Can you work these out from the model? Positions are in its coordinate system, mm. Face numbers are marked on the shaded views. A direction names the side the tool comes from. Give positions to 0.01 mm unless a question says otherwise; leave off trailing zeros. Order: outer loops, then holes, each group sorted by start corner. A loop starts at its lowest first (then second) coordinate and runs counter-clockwise, first axis right, second up. Notation, with made-up numbers: (-20.75, -23.75) - (1.25, -23.75) arc R23 ccw to (1.25, 11.25) - close; hole circle Ø1 at (-22.75, -39.5). An arc over 180 degrees is marked (long way). Use one line per item in the form item = value. Start each with the question number.
1) Please list where these lines run through material, in increasing order: probe 1 along Z at (x, y) = (17, 14); probe 2 along X at (y, z) = (9.5, 20); probe 3 along Z at (x, y) = (18.25, 18).
2) Suppose I cut it at B-B, the plane y = 11.25. Write out the boundary of the cut face in (x, z), and give its area (3 significant figures).
3) For pin 1 (3 mm diameter, centred on x = 12.5, y = 17, fed in from -Z); pin 2 (2 mm diameter, centred on x = 8.5, z = 16, fed in from +Y); pin 3 (2 mm diameter, centred on x = 8.5, y = 9.5, fed in from -Z), each with a flat end and sliding along its axis, tell me the tip position at first contact or that it passes through.
4) Suppose I cut it at A-A, the plane y = 2.5. Write out the boundary of the cut face in (x, z).
5) Suppose I cut it at D-D, the plane x = 17.5. Write out the boundary of the cut face in (y, z).
6) Suppose I cut it at C-C, the plane z = 17.5. Write out the boundary of the cut face in (x, y).
7) Which directions (+Z, -Z, +X, -X, +Y, -Y) give clear straight access to the entire face, cutting with the end or side of a thin tool? Please do the marked faces 4 and 5.
8) We'd pull the mould along X, two halves only. Please class the marked faces 1, 2 and 3: released by +X, released by -X, zero draft, split by the parting line, or undercut.
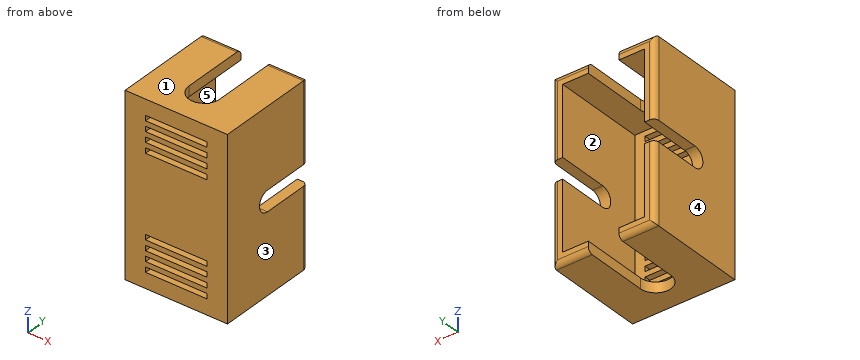
```python
from build123d import *

# Parameters (mm, degrees)
SKIZZE1_W                                   = 20
SKIZZE1_H                                   = 20
AUFSATZ_LINEAR_AUSTRAGEN1_DEPTH             = 35
WANDUNG1_T                                  = -2
SCHNITT_LINEAR_AUSTRAGEN2_DEPTH             = 33
VERRUNDUNG1_R                               = 1
SKIZZE4_W                                   = 12
SKIZZE4_H                                   = 1
SCHNITT_LINEAR_AUSTRAGEN3_DEPTH             = 2
LINEARES_MUSTER1_COUNT                      = 8
LINEARES_MUSTER1_PITCH                      = 2
LINEARES_MUSTER1_COL_COUNT                  = 8
LINEARES_MUSTER1_COL_PITCH                  = 2
SKIZZE5_W                                   = 12
SKIZZE5_H                                   = 15
AUFSATZ_LINEAR_AUSTRAGEN2_DEPTH             = 2
SCHNITT_LINEAR_AUSTRAGEN4_REACH             = 46.147
SCHNITT_LINEAR_AUSTRAGEN4_DIRECTION_2_REACH = 46.147


with BuildPart() as part:
    # Skizze1 → Aufsatz-Linear austragen1 (new body)
    with BuildSketch(Plane.XY):
        with Locations((10, 10)):
            Rectangle(SKIZZE1_W, SKIZZE1_H)
    extrude(amount=AUFSATZ_LINEAR_AUSTRAGEN1_DEPTH)

    # Wandung1
    wandung1_openings = [part.faces().sort_by_distance(p)[0] for p in [
        (10, 20, 17.5),
    ]]
    offset(amount=WANDUNG1_T, openings=wandung1_openings, kind=Kind.INTERSECTION)

    # Skizze3 → Schnitt-Linear austragen2 (cut)
    with BuildSketch(Plane.XY.offset(35)):
        with BuildLine():
            Line((13, 20), (13, 7))
            ThreePointArc((13, 7), (10, 4), (7, 7))
            Line((7, 7), (7, 20))
            ThreePointArc((7, 20), (10, 23), (13, 20))
        make_face()
    schnitt_linear_austragen2 = extrude(amount=-SCHNITT_LINEAR_AUSTRAGEN2_DEPTH, mode=Mode.SUBTRACT)

    # Spiegeln1: Schnitt-Linear austragen2 across plane
    add(schnitt_linear_austragen2.mirror(Plane.XY.offset(17.5)), mode=Mode.SUBTRACT)

    # Verrundung1
    verrundung1_edges = [part.edges().sort_by_distance(p)[0] for p in [
        (16.5, 20, 35),
        (3.5, 20, 35),
        (3.5, 20, 0),
        (16.5, 20, 0),
        (0, 20, 17.5),
        (20, 20, 17.5),
    ]]
    fillet(verrundung1_edges, radius=VERRUNDUNG1_R)

    # Skizze4 → Schnitt-Linear austragen3 (cut)
    with BuildSketch(Plane(origin=(0, 2, 0), x_dir=(1, 0, 0), z_dir=(0, 1, 0))):
        with Locations((10, -17.5)):
            Rectangle(SKIZZE4_W, SKIZZE4_H)
    schnitt_linear_austragen3 = extrude(amount=-SCHNITT_LINEAR_AUSTRAGEN3_DEPTH, mode=Mode.SUBTRACT)

    # Lineares Muster1: Schnitt-Linear austragen3 ×8
    with Locations(*[(0, 0, i * LINEARES_MUSTER1_PITCH) for i in range(1, LINEARES_MUSTER1_COUNT)]):
        add(schnitt_linear_austragen3, mode=Mode.SUBTRACT)

    # Lineares Muster1 col: Schnitt-Linear austragen3 ×8
    with Locations(*[(0, 0, -i * LINEARES_MUSTER1_COL_PITCH) for i in range(1, LINEARES_MUSTER1_COL_COUNT)]):
        add(schnitt_linear_austragen3, mode=Mode.SUBTRACT)

    # Skizze5 → Aufsatz-Linear austragen2 (add)
    with BuildSketch(Plane.XZ):
        with Locations((10, 17.5)):
            Rectangle(SKIZZE5_W, SKIZZE5_H)
    extrude(amount=-AUFSATZ_LINEAR_AUSTRAGEN2_DEPTH)

    # Schnitt-Linear austragen4: up to this face of the body (flat: up to its plane)
    schnitt_linear_austragen4_end = Plane(part.part.faces().sort_by_distance((20, 9.5, 17.5))[0])
    # Skizze7 → Schnitt-Linear austragen4 (cut, up to the picked face)
    with BuildSketch(Plane.ZY.offset(-18), mode=Mode.PRIVATE) as schnitt_linear_austragen4_sk1:
        with BuildLine():
            Line((19.5, 30), (19.5, 10))
            ThreePointArc((19.5, 10), (17.5, 8), (15.5, 10))
            Line((15.5, 10), (15.5, 30))
            ThreePointArc((15.5, 30), (17.5, 32), (19.5, 30))
        make_face()
    schnitt_linear_austragen4_tool1 = split(extrude(schnitt_linear_austragen4_sk1.sketch, amount=-SCHNITT_LINEAR_AUSTRAGEN4_REACH, mode=Mode.PRIVATE), bisect_by=schnitt_linear_austragen4_end, keep=Keep.BOTH, mode=Mode.PRIVATE)
    add(schnitt_linear_austragen4_tool1.solids().sort_by(Axis((18, 20, 17.5), (1, 0, 0)))[0], mode=Mode.SUBTRACT)

    # Schnitt-Linear austragen4 direction 2: up to this face of the body (flat: up to its plane)
    schnitt_linear_austragen4_direction_2_end = Plane(part.part.faces().sort_by_distance((0, 9.5, 17.5))[0])
    # Skizze7 → Schnitt-Linear austragen4 direction 2 (cut, up to the picked face)
    with BuildSketch(Plane.ZY.offset(-18), mode=Mode.PRIVATE) as schnitt_linear_austragen4_direction_2_sk1:
        with BuildLine():
            Line((19.5, 30), (19.5, 10))
            ThreePointArc((19.5, 10), (17.5, 8), (15.5, 10))
            Line((15.5, 10), (15.5, 30))
            ThreePointArc((15.5, 30), (17.5, 32), (19.5, 30))
        make_face()
    schnitt_linear_austragen4_direction_2_tool1 = split(extrude(schnitt_linear_austragen4_direction_2_sk1.sketch, amount=SCHNITT_LINEAR_AUSTRAGEN4_DIRECTION_2_REACH, mode=Mode.PRIVATE), bisect_by=schnitt_linear_austragen4_direction_2_end, keep=Keep.BOTH, mode=Mode.PRIVATE)
    add(schnitt_linear_austragen4_direction_2_tool1.solids().sort_by(Axis((18, 20, 17.5), (-1, 0, 0)))[0], mode=Mode.SUBTRACT)


solid = part.part
```
Result sheet:
q1.probe_1 = 0 to 2, 33 to 35
q1.probe_2 = 0 to 2, 18 to 20
q1.probe_3 = 0 to 15.5, 19.5 to 35
q2.outline = (0, 0) - (7, 0) - (7, 2) - (2, 2) - (2, 15.5) - (0, 15.5) - close; (0, 19.5) - (2, 19.5) - (2, 33) - (7, 33) - (7, 35) - (0, 35) - close; (13, 0) - (20, 0) - (20, 15.5) - (18, 15.5) - (18, 2) - (13, 2) - close; (13, 33) - (18, 33) - (18, 19.5) - (20, 19.5) - (20, 35) - (13, 35) - close
q2.area = 164 mm²
q3.pin_1 = 0
q3.pin_2 = 2
q3.pin_3 = through
q4.outline = (0, 0) - (20, 0) - (20, 35) - (0, 35) - close; hole (2, 2) - (18, 2) - (18, 33) - (2, 33) - close
q5.outline = (0, 0) - (19, 0) arc R1 ccw to (20, 1) - (20, 2) - (2, 2) - (2, 33) - (20, 33) - (20, 34) arc R1 ccw to (19, 35) - (0, 35) - close
q6.outline = (0, 0) - (20, 0) - (20, 8) - (18, 8) - (18, 2) - (2, 2) - (2, 8) - (0, 8) - close
q7.face_4 = +Z, -Z, -X, +Y, -Y
q7.face_5 = +Y
q8.face_1 = zero draft
q8.face_2 = undercut
q8.face_3 = released by +X
